For this review, take the finished solid that the model builds, in its own axes (mm). A direction names the side the tool comes from. Coordinates: 2 decimals unless noted, no trailing zeros. Order: outer loops, then holes, each group sorted by start corner. A loop starts at its lowest first (then second) coordinate and runs counter-clockwise, first axis right, second up. Notation, with made-up numbers: (83, -34) - (92, -34) arc R14 ccw to (92, -30) - close; hole circle Ø1 at (10.25, -12). An arc over 180 degrees is marked (long way). One line per item, written item: value. Start each with the question number.
(1) Clearance check with flat-ended pins moving along their axes: pin 1 (2 mm diameter, centred on y = 23.5, z = 5.5, fed in from +X); pin 2 (8 mm diameter, centred on x = 6, z = 6, fed in from +Y). State where each tip first meets the part, or that it passes through.
(2) Consider section B-B on y = 18.75. Write out the cut boundary in (x, z).
(3) Consider section A-A on z = 5.5. Write out the cut boundary in (x, y), then the cut area to 3 significant figures.
(4) Consider section C-C on z = 13.5. Write out the cut boundary in (x, y), then the cut area to 3 significant figures.
(5) Consider section D-D on z = 2. Write out the cut boundary in (x, y).
(6) To check wall thickness, follow line 1 along X through (y, z) = (5.25, 3.5); line 2 along X through (y, z) = (4.5, 6.75); line 3 along X through (y, z) = (10.25, 7.5). State the ranges of each line that lie inside material, in increasing order.
(7) Mouldability with a two-part tool opening along Z and no side actions: class faces 4 (the flat face through (-35.381, 3, 7)), 5 (the flat face through (-9, 10, 15.936)), 6 (the cylindrical face through (7.495, 3.131, 8.397)) as released by +Z, released by -Z, zero draft, split by the parting line, or undercut.
(8) For faces 1 (the flat face through (1.703, 12, 11)), 2 (the flat face through (17.959, 3, 7)), 3 (the flat face through (-19.125, 12, 11)), list the 3-axis set-ups (+Z, -Z, +X, -X, +Y, -Y) from which the entire face can be reached by the end or side of a thin tool; tool diameter is ignored.
```python
from build123d import *

# Parameters (mm, degrees)
SKETCH1_W           = 15.494
SKETCH1_H           = 19.05
SKETCH1_R           = 3.2639
SKETCH1_W_2         = 22.352
BOSS_EXTRUDE3_DEPTH = 6.35
SKETCH3_W           = 20.828
SKETCH3_H           = 19.05
BOSS_EXTRUDE4_DEPTH = 20.32
CUT_EXTRUDE1_REACH  = 39.084
SKETCH4_R           = 6.477


with BuildPart() as part:
    # Sketch1 → Boss-Extrude3 (new body)
    with BuildSketch(Plane(origin=(0, 0, 0), x_dir=(1, 0, 0), z_dir=(0, 1, 0))):
        with Locations((-27.634045528, -6.411090754)):
            Rectangle(SKETCH1_W, SKETCH1_H)
        with Locations((-27.507045528, -6.411090754)):
            Circle(SKETCH1_R, mode=Mode.SUBTRACT)
        with Locations((-8.711045528, -6.411090754)):
            Rectangle(SKETCH1_W_2, SKETCH1_H)
        with Locations((10.211954472, -6.411090754)):
            Rectangle(SKETCH1_W, SKETCH1_H)
        with Locations((10.084954472, -6.411090754)):
            Circle(SKETCH1_R, mode=Mode.SUBTRACT)
    extrude(amount=BOSS_EXTRUDE3_DEPTH)

    # Sketch3 → Boss-Extrude4 (add)
    with BuildSketch(Plane(origin=(0, 6.35, 0), x_dir=(1, 0, 0), z_dir=(0, 1, 0))):
        with Locations((-8.711045528, -6.411090754)):
            Rectangle(SKETCH3_W, SKETCH3_H)
    extrude(amount=BOSS_EXTRUDE4_DEPTH)

    # Sketch4 → Cut-Extrude1 (cut, up to next)
    with BuildSketch(Plane.ZY.offset(19.125045528), mode=Mode.PRIVATE) as cut_extrude1_sk1:
        with Locations((6.411090754, 17.656309415)):
            Circle(SKETCH4_R)
    cut_extrude1_tool1 = extrude(cut_extrude1_sk1.sketch, amount=-CUT_EXTRUDE1_REACH, mode=Mode.PRIVATE) & part.part
    add(cut_extrude1_tool1.solids().sort_by_distance((-19.125046, 17.656309, 6.411091))[0], mode=Mode.SUBTRACT)


solid = part.part
```
Geometry check:
1. pin 1: stops at x = 1.7
1. pin 2: stops at y = 6.35
2. outline: (-19.13, -3.11) - (1.7, -3.11) - (1.7, 0.03) - (-19.13, 0.03) - close; (-19.13, 12.8) - (1.7, 12.8) - (1.7, 15.94) - (-19.13, 15.94) - close
3. outline: (-35.38, 0) - (-30.64, 0) - (-30.64, 6.35) - (-35.38, 6.35) - close; (-24.37, 0) - (6.95, 0) - (6.95, 6.35) - (1.7, 6.35) - (1.7, 11.24) - (-19.13, 11.24) - (-19.13, 6.35) - (-24.37, 6.35) - close; (-19.13, 24.07) - (1.7, 24.07) - (1.7, 26.67) - (-19.13, 26.67) - close; (13.22, 0) - (17.96, 0) - (17.96, 6.35) - (13.22, 6.35) - close
3. area: 415 mm^2
4. outline: (-35.38, 0) - (17.96, 0) - (17.96, 6.35) - (1.7, 6.35) - (1.7, 26.67) - (-19.13, 26.67) - (-19.13, 6.35) - (-35.38, 6.35) - close
4. area: 762 mm^2
5. outline: (-35.38, 0) - (17.96, 0) - (17.96, 6.35) - (1.7, 6.35) - (1.7, 12.91) - (-19.13, 12.91) - (-19.13, 6.35) - (-35.38, 6.35) - close; (-19.13, 22.4) - (1.7, 22.4) - (1.7, 26.67) - (-19.13, 26.67) - close
6. line 1: x = -35.38 to -28.98, -26.03 to 8.61, 11.56 to 17.96
6. line 2: x = -35.38 to -30.75, -24.26 to 6.84, 13.33 to 17.96
6. line 3: x = -19.13 to 1.7
7. face 4: zero draft
7. face 5: released by +Z
7. face 6: undercut
8. face 1: +Z, -Z, +X, +Y
8. face 2: +Z, -Z, +X, +Y, -Y
8. face 3: +Z, -Z, -X, +Y
